Model file for the job. Use its own axes, mm. A direction names the side the tool comes from. Give positions to 0.01 mm unless a question says otherwise; leave off trailing zeros. Write each loop counter-clockwise with the first axis right and the second up, starting at its lowest first coordinate (ties: lowest second). Pieces come first, ordered by that corner, then holes.
```python
from build123d import *

# Parameters (mm, degrees)
SALIENTE_EXTRUIR1_DEPTH = 90
CORTAR_EXTRUIR1_REACH   = 124.984
CROQUIS3_R              = 5


with BuildPart() as part:
    # Croquis2 → Saliente-Extruir1 (new body)
    with BuildSketch(Plane.XY):
        Polygon((0, 0), (0, 25), (-80, 25), (-80, 0), (-60, 0), (-60, 6), (-20, 6), (-20, 0), align=None)
    extrude(amount=-SALIENTE_EXTRUIR1_DEPTH)

    # Croquis3 → Cortar-Extruir1 (cut, up to next)
    with BuildSketch(Plane(origin=(0, 25, 0), x_dir=(1, 0, 0), z_dir=(0, 1, 0)), mode=Mode.PRIVATE) as cortar_extruir1_sk1:
        with Locations(Location((-70, 80, 0), (0, 0, 180))):
            Circle(CROQUIS3_R)
    cortar_extruir1_tool1 = extrude(cortar_extruir1_sk1.sketch, amount=-CORTAR_EXTRUIR1_REACH, mode=Mode.PRIVATE) & part.part
    # Croquis3 → Cortar-Extruir1 (cut, up to next)
    with BuildSketch(Plane(origin=(0, 25, 0), x_dir=(1, 0, 0), z_dir=(0, 1, 0)), mode=Mode.PRIVATE) as cortar_extruir1_sk2:
        with Locations(Location((-10, 80, 0), (0, 0, 180))):
            Circle(CROQUIS3_R)
    cortar_extruir1_tool2 = extrude(cortar_extruir1_sk2.sketch, amount=-CORTAR_EXTRUIR1_REACH, mode=Mode.PRIVATE) & part.part
    # Croquis3 → Cortar-Extruir1 (cut, up to next)
    with BuildSketch(Plane(origin=(0, 25, 0), x_dir=(1, 0, 0), z_dir=(0, 1, 0)), mode=Mode.PRIVATE) as cortar_extruir1_sk3:
        with Locations(Location((-10, 10, 0), (0, 0, 180))):
            Circle(CROQUIS3_R)
    cortar_extruir1_tool3 = extrude(cortar_extruir1_sk3.sketch, amount=-CORTAR_EXTRUIR1_REACH, mode=Mode.PRIVATE) & part.part
    # Croquis3 → Cortar-Extruir1 (cut, up to next)
    with BuildSketch(Plane(origin=(0, 25, 0), x_dir=(1, 0, 0), z_dir=(0, 1, 0)), mode=Mode.PRIVATE) as cortar_extruir1_sk4:
        with Locations(Location((-70, 10, 0), (0, 0, 180))):
            Circle(CROQUIS3_R)
    cortar_extruir1_tool4 = extrude(cortar_extruir1_sk4.sketch, amount=-CORTAR_EXTRUIR1_REACH, mode=Mode.PRIVATE) & part.part
    add(cortar_extruir1_tool1.solids().sort_by_distance((-70, 25, -80))[0], mode=Mode.SUBTRACT)
    add(cortar_extruir1_tool2.solids().sort_by_distance((-10, 25, -80))[0], mode=Mode.SUBTRACT)
    add(cortar_extruir1_tool3.solids().sort_by_distance((-10, 25, -10))[0], mode=Mode.SUBTRACT)
    add(cortar_extruir1_tool4.solids().sort_by_distance((-70, 25, -10))[0], mode=Mode.SUBTRACT)

    # Croquis5 → Recubrir1 section 0
    with BuildSketch(Plane.ZY.offset(80)):
        with BuildLine():
            Line((-72.5, 25), (-47.5, 25))
            ThreePointArc((-47.5, 25), (-60, 37.5), (-72.5, 25))
        make_face()
    # Croquis4 → Recubrir1 section 1
    with BuildSketch(Plane(origin=(0, 0, 0), x_dir=(0, 0, -1), z_dir=(1, 0, 0))):
        with BuildLine():
            Line((42.5, 25), (17.5, 25))
            ThreePointArc((17.5, 25), (30, 37.5), (42.5, 25))
        make_face()
    loft()

    # Cortar-Recubrir1: read off the stored shape, not the designer's step
    # Cortar-Recubrir1: loft between two sections, ruled curve by curve
    cortar_recubrir1_from = [
        Edge.make_bspline([(-80, 27.8178005, -66.950539572), (-80, 28.397012131, -66.715722864), (-80, 29.023662616, -66.379666069), (-80, 29.965028032, -65.63546774), (-80, 30.27819737, -65.347207423), (-80, 30.878995513, -64.678611595), (-80, 31.166580719, -64.298055634), (-80, 31.682547567, -63.441447082), (-80, 31.910716085, -62.965172363), (-80, 32.268300366, -61.929262486), (-80, 32.397319654, -61.369555656), (-80, 32.520385943, -60.19953953), (-80, 32.51399771, -59.589467861), (-80, 32.346580783, -58.370138344), (-80, 32.18535628, -57.761411131), (-80, 31.715722864, -56.602987869), (-80, 31.407536262, -56.053840186), (-80, 30.678592509, -55.062157825), (-80, 30.258345404, -54.619867625), (-80, 29.355265136, -53.865858955), (-80, 28.87290981, -53.554007946), (-80, 27.894905327, -53.059555699), (-80, 27.399490807, -52.876626932), (-80, 26.43267588, -52.621149153), (-80, 25.961273747, -52.548292311), (-80, 25.064501609, -52.486822627), (-80, 24.639009381, -52.49802121), (-80, 23.44516904, -52.619451193), (-80, 22.761411131, -52.81464372), (-80, 21.602987869, -53.284277136), (-80, 20.976337384, -53.620333931), (-80, 20.034971968, -54.36453226), (-80, 19.72180263, -54.652792577), (-80, 19.121004487, -55.321388405), (-80, 18.833419281, -55.701944366), (-80, 18.317452433, -56.558552918), (-80, 18.089283915, -57.034827637), (-80, 17.731699634, -58.070737514), (-80, 17.602680346, -58.630444344), (-80, 17.479614057, -59.80046047), (-80, 17.48600229, -60.410532139), (-80, 17.653419217, -61.629861656), (-80, 17.81464372, -62.238588869), (-80, 18.284277136, -63.397012131), (-80, 18.592463738, -63.946159814), (-80, 19.321407491, -64.937842175), (-80, 19.741654596, -65.380132375), (-80, 20.644734864, -66.134141045), (-80, 21.12709019, -66.445992054), (-80, 22.105094673, -66.940444301), (-80, 22.600509193, -67.123373068), (-80, 23.56732412, -67.378850847), (-80, 24.038726253, -67.451707689), (-80, 24.935498391, -67.513177373), (-80, 25.360990619, -67.50197879), (-80, 26.55483096, -67.380548807), (-80, 27.238588869, -67.18535628), (-80, 27.8178005, -66.950539572)], [0, 0, 0, 0, 0.0625, 0.0625, 0.09375, 0.09375, 0.125, 0.125, 0.15625, 0.15625, 0.1875, 0.1875, 0.21875, 0.21875, 0.25, 0.25, 0.28125, 0.28125, 0.3125, 0.3125, 0.34375, 0.34375, 0.375, 0.375, 0.40625, 0.40625, 0.4375, 0.4375, 0.5, 0.5, 0.5625, 0.5625, 0.59375, 0.59375, 0.625, 0.625, 0.65625, 0.65625, 0.6875, 0.6875, 0.71875, 0.71875, 0.75, 0.75, 0.78125, 0.78125, 0.8125, 0.8125, 0.84375, 0.84375, 0.875, 0.875, 0.90625, 0.90625, 0.9375, 0.9375, 1, 1, 1, 1], 3),
    ]
    cortar_recubrir1_to = [
        Edge.make_bspline([(0, 31.377503921, -33.946827047), (0, 31.706406175, -33.415368387), (0, 32.013835032, -32.774187836), (0, 32.33435549, -31.617785382), (0, 32.416968296, -31.200239973), (0, 32.507224255, -30.305906337), (0, 32.514702079, -29.828965909), (0, 32.425496651, -28.83295266), (0, 32.328510244, -28.313826359), (0, 32.005617859, -27.266584123), (0, 31.779349551, -26.738644387), (0, 31.187995987, -25.721597678), (0, 30.822699703, -25.232939438), (0, 29.967766964, -24.347567814), (0, 29.478285707, -23.951398333), (0, 28.415368387, -23.293593825), (0, 27.84243548, -23.032270186), (0, 26.668642711, -22.662130437), (0, 26.06833886, -22.553210568), (0, 24.894293414, -22.477709998), (0, 24.320859272, -22.510740236), (0, 23.239559888, -22.688974452), (0, 22.73169069, -22.833775549), (0, 21.800495492, -23.198296471), (0, 21.37698638, -23.417768843), (0, 20.616854994, -23.897538648), (0, 20.280022745, -24.15775602), (0, 19.388077935, -24.960522771), (0, 18.951398333, -25.521714293), (0, 18.293593825, -26.584631613), (0, 17.986164968, -27.225812164), (0, 17.66564451, -28.382214618), (0, 17.583031704, -28.799760027), (0, 17.492775745, -29.694093663), (0, 17.485297921, -30.171034091), (0, 17.574503349, -31.16704734), (0, 17.671489756, -31.686173641), (0, 17.994382141, -32.733415877), (0, 18.220650449, -33.261355613), (0, 18.812004013, -34.278402322), (0, 19.177300297, -34.767060562), (0, 20.032233036, -35.652432186), (0, 20.521714293, -36.048601667), (0, 21.584631613, -36.706406175), (0, 22.15756452, -36.967729814), (0, 23.331357289, -37.337869563), (0, 23.93166114, -37.446789432), (0, 25.105706586, -37.522290002), (0, 25.679140728, -37.489259764), (0, 26.760440112, -37.311025548), (0, 27.26830931, -37.166224451), (0, 28.199504508, -36.801703529), (0, 28.62301362, -36.582231157), (0, 29.383145006, -36.102461352), (0, 29.719977255, -35.84224398), (0, 30.611922065, -35.039477229), (0, 31.048601667, -34.478285707), (0, 31.377503921, -33.946827047)], [0, 0, 0, 0, 0.0625, 0.0625, 0.09375, 0.09375, 0.125, 0.125, 0.15625, 0.15625, 0.1875, 0.1875, 0.21875, 0.21875, 0.25, 0.25, 0.28125, 0.28125, 0.3125, 0.3125, 0.34375, 0.34375, 0.375, 0.375, 0.40625, 0.40625, 0.4375, 0.4375, 0.5, 0.5, 0.5625, 0.5625, 0.59375, 0.59375, 0.625, 0.625, 0.65625, 0.65625, 0.6875, 0.6875, 0.71875, 0.71875, 0.75, 0.75, 0.78125, 0.78125, 0.8125, 0.8125, 0.84375, 0.84375, 0.875, 0.875, 0.90625, 0.90625, 0.9375, 0.9375, 1, 1, 1, 1], 3),
    ]
    cortar_recubrir1 = Solid(Shell([*[Face.make_surface_from_curves(cortar_recubrir1_from[k], cortar_recubrir1_to[k]) for k in range(1)], Face(Wire(cortar_recubrir1_from)), Face(Wire(cortar_recubrir1_to))]))
    add(cortar_recubrir1, mode=Mode.SUBTRACT)


solid = part.part
```
1. Pin check, flat tips, straight feed: P1, Ø3, axis at x = -48.5, z = -28, coming from the +Y side; P2, Ø6, axis at x = -10, z = -80, coming from the +Y side; P3, Ø14.5, axis at x = -38, z = -60.5, coming from the +Y side. Stop position of each tip, or through.
Calculated:
P1: stops at y = 25
P2: passes through
P3: stops at y = 34.16
2. Slice it at C-C, the plane x = -70. State how many separate pieces and enclosed holes the cut face has, and give its area (3 significant figures).
Calculated:
separate pieces: 3
enclosed holes: 1
area: 1,830 mm2
3. Slice it at B-B, the plane z = -80. Write the cut outline in (x, y), and give its area (3 significant figures).
Calculated:
outline: (-80, 0) - (-75, 0) - (-75, 25) - (-80, 25) - close; (-65, 0) - (-60, 0) - (-60, 6) - (-20, 6) - (-20, 0) - (-15, 0) - (-15, 25) - (-65, 25) - close; (-5, 0) - (0, 0) - (0, 25) - (-5, 25) - close
area: 1,260 mm2
4. Pull direction X, two halves, no side cores. Call faces 6 (the cylindrical face through (-14.77, 12.68, -8.5)), 7 (the flat face through (-10, 0, -44)), 8 (the cylindrical face through (-8.92, 12.68, -84.88)), 9 (the flat face through (-80, 15, -44)): +X half, -X half, draft (parallel to the pull), parting line (faces both ways), or undercut.
Calculated:
face 6: undercut
face 7: draft
face 8: undercut
face 9: -X half
5. Which spindle directions (+Z, -Z, +X, -X, +Y, -Y) get a long thin tool onto all of the face, cutting with end or side? Do faces 1 (the flat face through (-41, 13, -90)), 2 (the flat face through (-48, 25, -18)), 3 (the flat face through (-31, 25, -71)), 4 (the flat face through (-60, 3, -44)), 5 (the cylindrical face through (-74.619, 12.675, -11.915)). Say none if no direction does.
Calculated:
face 1: -Z, +X, -X, +Y, -Y
face 2: +Z, -X, +Y
face 3: -Z, +X, +Y
face 4: +Z, -Z, -Y
face 5: +Y, -Y
6. Probe probe 1 along Z at (x, y) = (-70, 12); probe 2 along X at (y, z) = (13, -6); probe 3 along Z at (x, y) = (-68, 24.5). List the from-to ranges inside material, lowest first.
Calculated:
probe 1: z = -90 to -85, -75 to -15, -5 to 0
probe 2: x = -80 to -73, -67 to -13, -7 to 0
probe 3: z = -90 to -84.58, -75.42 to -62.8, -48.2 to -14.58, -5.42 to 0
7. Slice it at A-A, the plane y = 12.5. Write the cut outline in (x, z).
Calculated:
outline: (-80, -90) - (0, -90) - (0, 0) - (-80, 0) - close; hole circle Ø10 at (-70, -80); hole circle Ø10 at (-70, -10); hole circle Ø10 at (-10, -80); hole circle Ø10 at (-10, -10)
